from build123d import *

# Parameters (mm, degrees)
SKETCH1_W           = 180
SKETCH1_H           = 180
BOSS_EXTRUDE1_DEPTH = 5
CUT_EXTRUDE1_DEPTH  = 128.377392029


with BuildPart() as part:
    # Sketch1 → Boss-Extrude1 (new body)
    with BuildSketch(Plane.XY):
        Rectangle(SKETCH1_W, SKETCH1_H)
    extrude(amount=BOSS_EXTRUDE1_DEPTH)

    # Sketch3 → Cut-Extrude1 (cut, through all)
    with BuildSketch(Plane(origin=(0, 0, 0), x_dir=(-1, 0, 0), z_dir=(0, 0, -1))):
        with BuildLine():
            Line((-34.154155691, -13.446054827), (23.801393887, 2.083087879))
            ThreePointArc((23.801393887, 2.083087879), (48.296291314, -12.059047745), (34.154155691, -36.553945173))
            Line((34.154155691, -36.553945173), (-23.801393887, -52.083087879))
            ThreePointArc((-23.801393887, -52.083087879), (-48.296291314, -37.940952255), (-34.154155691, -13.446054827))
        make_face()
    extrude(amount=-CUT_EXTRUDE1_DEPTH, mode=Mode.SUBTRACT)


solid = part.part
Can you work these out from the model? Positions are in its coordinate system, mm. A direction names the side the tool comes from. Round coordinates to 2 decimals unless told otherwise and drop trailing zeros. Write each loop counter-clockwise with the first axis right and the second up, starting at its lowest first coordinate (ties: lowest second). Pieces come first, ordered by that corner, then holes. Notation, with made-up numbers: (84, -2.75) -> (104, -2.75) arc R25 cw to (104, 14.25) -> close; hole circle Ø1 at (75, 5). An arc over 180 degrees is marked (long way). Use one line per item in the form item = value. Start each with the question number.
Q1. If I drill on probe 1 along Y at (x, z) = (-4.5, 3.5); probe 2 along Y at (x, z) = (-3, 3.15); probe 3 along X at (y, z) = (-24, 0.9), over which ranges is the centre line in solid material (lowest first)? Write a range as [from, to].
Q2. Imagine slicing it at A-A (x = 11). Please give me the cut outline in (y, z).
Q3. Imagine slicing it at B-B (z = 2.8). Please give me the cut outline in (x, y), then the cut area to 3 significant figures.
Q4. Imagine slicing it at C-C (y = -49). Please give me the cut outline in (x, z), then the cut area to 3 significant figures.
Q5. Which directions (+Z, -Z, +X, -X, +Y, -Y) give clear straight access to the entire face, cutting with the end or side of a thin tool? Please do faces 5 (the face through (-90, -1, 2)), 6 (the face through (-5.58, -44.21, 2.46)).
Q6. We'd pull the mould along X, two halves only. Please class faces 1 (the face through (-48.18, -11.64, 2.46)), 2 (the face through (-1, -90, 2)), 3 (the face through (90, -1, 2)), 4 (the face through (48.18, -38.36, 2.46)): +X half, -X half, draft (parallel to the pull), parting line (faces both ways), or undercut.
Worked out:
q1.probe_1 = [-90, -44.5], [-3.09, 90]
q1.probe_2 = [-90, -44.9], [-3.49, 90]
q1.probe_3 = [-90, -47.8], [46.96, 90]
q2.outline = (-90, 0) -> (-48.65, 0) -> (-48.65, 5) -> (-90, 5) -> close; (-7.24, 0) -> (90, 0) -> (90, 5) -> (-7.24, 5) -> close
q3.outline = (-90, -90) -> (90, -90) -> (90, 90) -> (-90, 90) -> close; hole (-34.15, -36.55) -> (23.8, -52.08) arc R20 ccw to (34.15, -13.45) -> (-23.8, 2.08) arc R20 ccw to start
q3.area = 28,700 mm^2
q4.outline = (-90, 0) -> (12.3, 0) -> (12.3, 5) -> (-90, 5) -> close; (40.66, 0) -> (90, 0) -> (90, 5) -> (40.66, 5) -> close
q4.area = 758 mm^2
q5.face_5 = +Z, -Z, -X, +Y, -Y
q5.face_6 = +Z, -Z
q6.face_1 = undercut
q6.face_2 = draft
q6.face_3 = +X half
q6.face_4 = undercut
